Autodesk Inventor part; units mm, degrees
ref_plane "YZ Plane" through (0, 0, 0) normal (1, 0, 0) x (0, 1, 0)
ref_plane "XZ Plane" through (0, 0, 0) normal (0, 1, 0) x (-1, 0, 0)
ref_plane "XY Plane" through (0, 0, 0) normal (0, 0, 1) x (1, 0, 0)
sketch "Sketch1" plane through (0, 0, 0) normal (0, 0, 1) x (1, 0, 0)
  line L0 (5, -10) -> (-5, -10)
  line L1 (-5, -10) -> (-5, 10)
  line L2 (-5, 10) -> (5, 10)
  line L3 (5, 10) -> (5, -10)
  line L4 (5, -10) -> (-5, 10) construction
  line L5 (-5, -10) -> (5, 10) construction
  point P0 (0, 0)
  dimension "d0" = 10
  dimension "d1" = 20
extrude "Extrusion1" add sketch "Sketch1" along normal blind 2
sketch "Sketch2" plane through (0, 0, 0) normal (0, 0, -1) x (-1, 0, 0)
  line L0 (-5, -10) -> (5, -10) construction
  line L1 (5, -10) -> (5, 10) construction
  line L2 (5, 10) -> (-5, 10) construction
  line L3 (-5, 10) -> (-5, -10) construction
  line L4 (-5, -10) -> (-5, 10)
  line L5 (-5, 10) -> (-10, 10)
  line L6 (-10, 10) -> (-10, -10)
  line L7 (-10, -10) -> (-5, -10)
  line L8 (-5, -10) -> (-5, 10)
  line L9 (5, 10) -> (5, -10)
  line L10 (5, 10) -> (10, 10)
  line L11 (10, 10) -> (10, -10)
  line L12 (10, -10) -> (5, -10)
  line L13 (5, -10) -> (5, 10)
  line L14 (5, -10) -> (-5, -10)
  point P0 (0, 0)
  dimension "d4" = 5
  dimension "d5" = 5
extrude "Extrusion2" add sketch "Sketch2" against normal blind 10
sketch "Sketch3" plane through (-10, 10, 0) normal (0, 1, 0) x (1, 0, 0)
  line L0 (0, 0) -> (20, 0) construction
  line L1 (0, 0) -> (0, -10) construction
  line L2 (5, -10) -> (0, -10) construction
  line L3 (5, -2) -> (5, -10) construction
  line L4 (15, -2) -> (5, -2) construction
  line L5 (15, -2) -> (15, -10) construction
  line L6 (20, -10) -> (15, -10) construction
  line L7 (20, 0) -> (20, -10) construction
  line L8 (5, -8) -> (1.6755, -2.3008)
  line L9 (1.8482, -2) -> (5, -2)
  line L10 (15, -8) -> (18.3245, -2.3008)
  line L11 (18.1518, -2) -> (15, -2)
  arc A0 (1.8482, -2) -> (1.6755, -2.3008) centre (1.8482, -2.2) ccw
  arc A1 (18.3245, -2.3008) -> (18.1518, -2) centre (18.1518, -2.2) ccw
  line L12 (5, -2) -> (5, -10)
  line L13 (5, -8) -> (5, -2)
  line L14 (15, -2) -> (15, -8)
  line L15 (15, -2) -> (15, -10)
  point P0 (10, 0)
  point P1 (1.5, -2)
  point P2 (18.5, -2)
  dimension "d9" = 2
  dimension "d10" = 3.5
  dimension "d11" = 3.5
  dimension "d12" = 2
  dimension "d13" = 0.2
extrude "Extrusion3" cut sketch "Sketch3" against normal through all
sketch "Sketch4" plane through (-10, 10, 0) normal (0, 1, 0) x (1, 0, 0)
  line L0 (0, -3.3978) -> (3.2724, -9.0077)
  line L1 (5, -10) -> (0, -10)
  line L2 (5, -8) -> (1.6755, -2.3008)
  line L3 (1.8482, -2) -> (18.1518, -2)
  line L4 (0, 0) -> (20, 0)
  line L5 (0, 0) -> (0, -10)
  line L6 (0, -3.3978) -> (0, -10)
  line L7 (20, -3.3381) -> (16.7016, -8.9926)
  line L8 (20, -10) -> (15, -10)
  line L9 (18.3245, -2.3008) -> (15, -8)
  line L10 (20, 0) -> (20, -10)
  line L11 (20, -3.3381) -> (20, -10)
  line L12 (5, -8) -> (3.2724, -9.0077)
  line L13 (15, -8) -> (15, -10)
  line L14 (15, -8) -> (16.7016, -8.9926)
  line L15 (5, -8) -> (5, -10)
  line L16 (5, -8) -> (5, -10)
  point P0 (10, 0)
  dimension "d16" = 2
  dimension "d17" = 2
extrude "Extrusion4" cut sketch "Sketch4" against normal through all
sketch "Sketch6" plane through (-10, -10, 0) normal (0, -1, 0) x (1, 0, 0)
  line L0 (1.6755, 2.3008) -> (5, 8)
  line L1 (18.1518, 2) -> (1.8482, 2)
  line L2 (15, 8) -> (18.3245, 2.3008)
  arc A0 (18.1518, 2) -> (18.3245, 2.3008) centre (18.1518, 2.2) ccw
  arc A1 (1.6755, 2.3008) -> (1.8482, 2) centre (1.8482, 2.2) ccw
  line L3 (3.2724, 9.0077) -> (5, 8)
  line L4 (5, 8) -> (15, 8)
  point P0 (10, 0)
extrude "Extrusion6" add sketch "Sketch6" against normal blind 2
fillet "Fillet1" [suppressed]
fillet "Fillet2" radius 1 4 edges at (6.7016, 0, 8.9926) (-10, 0, 0) (10, 0, 0) (-6.7276, 0, 9.0077)
equation "\"d12\" = d9"
properties part number "rail"
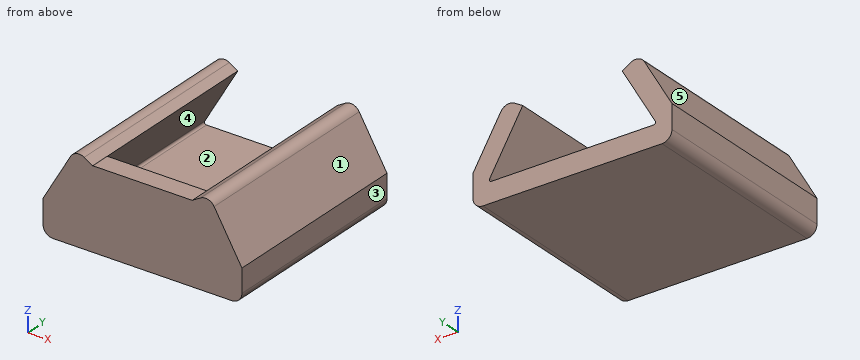
The listing builds one solid part. Answer for the finished solid, in the listing's coordinates (mm). Face numbers are marked on the shaded views. A direction names the side the tool comes from. Round coordinates to 2 decimals unless told otherwise and drop trailing zeros. Order: outer loops, then holes, each group sorted by start corner. A loop starts at its lowest first (then second) coordinate and runs counter-clockwise, first axis right, second up. Notation, with made-up numbers: M -40,60.5 L -23,60.5 A13 cw -23,81.5 Z; hole C 56,-15 d9. An arc over 180 degrees is marked long. Answer in a Markdown table with one row per item. Add a question column.
1) Flat-ended cylindrical pins translate along their axes: pin 1 Ø3 at (x, y) = (1, -2.5) entering from +Z; pin 2 Ø5 at (x, y) = (3.5, -2.5) entering from +Z; pin 3 Ø0.6 at (x, y) = (0.5, -9.5) entering from +Z. Find the tip coordinate at first contact, or state that the pin passes through.
2) The part is cut by section C-C on z = 7.25. Determine the outline of the cut face in (x, y), plus the area to 3 significant figures.
3) The part is cut by section A-A on y = -1.75. Determine the outline of the cut face in (x, z), plus the area to 3 significant figures.
4) Determine the mould class of the marked faces 1, 2 and 3 for opening direction Z: pulls with the +Z half, pulls with the -Z half, needs draft (parallel to the pull), parting line crosses it, or undercut.
5) The part is cut by section B-B on x = 4. Determine the outline of the cut face in (y, z).
6) Consider line 1 along Y through (x, z) = (1.5, 3.5); line 2 along X through (y, z) = (7.5, 7.5); line 3 along X through (y, z) = (-4, 5.25). Determine where each line is inside the solid, lowest interval first. Write a range as from..to.
7) Which of the six approach directions +Z, -Z, +X, -X, +Y, -Y give full straight-line access (tool end or side, diameter ignored) to the marked faces 4 and 5?
8) The part is cut by section D-D on y = -8.5. Determine the outline of the cut face in (x, z), plus the area to 3 significant figures.
Findings below:
| question | item | result |
|---|---|---|
| 1 | pin 1 | stops at z = 2 |
| 1 | pin 2 | stops at z = 8.56 |
| 1 | pin 3 | stops at z = 8 |
| 2 | outline | M -7.75,-10 L 7.72,-10 L 7.72,10 L 5.44,10 L 5.44,-8 L -5.44,-8 L -5.44,10 L -7.75,10 Z |
| 2 | area | 114 mm² |
| 3 | outline | M -10,1 A1 ccw -9,0 L 9,0 A1 ccw 10,1 L 10,3.34 L 7.21,8.13 A1 ccw 5.84,8.49 L 5,8 L 8.32,2.3 A0.2 cw 8.15,2 L -8.15,2 A0.2 cw -8.32,2.3 L -5,8 L -5.86,8.5 A1 ccw -7.23,8.14 L -10,3.4 Z |
| 3 | area | 68.0 mm² |
| 4 | face 1 | pulls with the +Z half |
| 4 | face 2 | undercut |
| 4 | face 3 | needs draft |
| 5 | outline | M -10,0 L 10,0 L 10,2 L -8,2 L -8,8 L -10,8 Z |
| 6 | line 1 | y = -10..-8 |
| 6 | line 2 | x = -7.61..-5.29, 5.29..7.57 |
| 6 | line 3 | x = -8.92..-6.6, 6.6..8.88 |
| 7 | face 4 | +Y |
| 7 | face 5 | +Z, -X, +Y, -Y |
| 8 | outline | M -10,1 A1 ccw -9,0 L 9,0 A1 ccw 10,1 L 10,3.34 L 7.21,8.13 A1 ccw 5.84,8.49 L 5,8 L -5,8 L -5.86,8.5 A1 ccw -7.23,8.14 L -10,3.4 Z |
| 8 | area | 149 mm² |
